Can you work these out from the model? Positions are in its coordinate system, mm. A direction names the side the tool comes from. Give positions to 0.01 mm unless a question says otherwise; leave off trailing zeros. Order: outer loops, then holes, each group sorted by start corner. A loop starts at its lowest first (then second) coordinate and runs counter-clockwise, first axis right, second up. Notation, with made-up numbers: M 34,42 L 84,42 A18 ccw 84,71 Z; hole C 72.25,-2.75 d9. An arc over 180 degrees is marked long. Write each question's results on one line, items separated by ' | '.
from build123d import *

# Parameters (mm, degrees)
CUT_EXTRUDE1_DEPTH = 1.41097
SKETCH5_R          = 1.833087105
CUT_EXTRUDE2_DEPTH = 1.41097
CUT_EXTRUDE2_DRAFT = -60
FILLET1_R          = 0.12827


with BuildPart() as part:
    # Sketch3 → Revolve1 (revolve)
    with BuildSketch(Plane(origin=(0, 0, 0), x_dir=(0, 0, -1), z_dir=(1, 0, 0))):
        with BuildLine():
            Line((-6.83895, 0), (-6.83895, 2.2225))
            ThreePointArc((-6.83895, 2.2225), (-5.93321038, 3.573966445), (-4.65836, 4.5847))
            Line((-4.65836, 4.5847), (-4.27355, 4.516847615))
            Line((-4.27355, 4.516847615), (-4.27355, 2.413))
            Line((-4.27355, 2.413), (6.2436375, 2.413))
            Line((6.2436375, 2.413), (6.83895, 1.8176875))
            Line((6.83895, 1.8176875), (6.83895, 0))
            Line((6.83895, 0), (-6.83895, 0))
        make_face()
    revolve(axis=Axis((0, 0, 6.83895), (0, 0, -1)))

    # Sketch4 → Cut-Extrude1 (cut)
    with BuildSketch(Plane.XY.offset(6.83895)):
        Polygon((-1.5875, -0.916543552), (0, -1.833087105), (1.5875, -0.916543552), (1.5875, 0.916543552), (0, 1.833087105), (-1.5875, 0.916543552), align=None)
    extrude(amount=-CUT_EXTRUDE1_DEPTH, mode=Mode.SUBTRACT)


with BuildPart() as cut_extrude2_tool:
    # Sketch5 → Cut-Extrude2 (with draft: the straight prism first)
    with BuildSketch(Plane.XY.offset(6.83895)):
        Circle(SKETCH5_R)
    extrude(amount=-CUT_EXTRUDE2_DEPTH)
    # Cut-Extrude2: the draft: its side faces are tilted about the plane it starts from
    cut_extrude2_sides = [cut_extrude2_tool.faces().sort_by_distance(p)[0] for p in [
        (-1.833087105, 0, 6.133465),
    ]]
    draft(cut_extrude2_sides, Plane.XY.offset(6.83895), CUT_EXTRUDE2_DRAFT)


with BuildPart() as part_1:
    add(part.part)

    # Cut-Extrude2: cut by cut_extrude2_tool
    add(cut_extrude2_tool.part, mode=Mode.SUBTRACT)

    # Fillet1
    fillet1_edges = [part_1.edges().sort_by_distance(p)[0] for p in [
        (0, -4.516847615, 4.27355),
        (0, -4.5847, 4.65836),
    ]]
    fillet(fillet1_edges, radius=FILLET1_R)


solid = part_1.part
(1) Imagine slicing it at B-B, the plane z = -1. Write out the boundary of the cut face in (x, y), plus the area to 3 significant figures.
Data:
outline: C 0,0 d4.83 | area: 18.3 mm2
(2) We'd pull the mould along Y, two halves only. Please class faces 1 (the face through (-1.588, 0, 6)), 2 (the face through (2, 0, 6.839)), 3 (the face through (-1.468, -1.915, -1.059)): +Y half, -Y half, draft (parallel to the pull), parting line (faces both ways), or undercut.
Data:
face 1: undercut | face 2: draft | face 3: parting line
(3) Imagine slicing it at A-A, the plane z = 5.75. Write out the boundary of the cut face in (x, y), plus the area to 3 significant figures.
Data:
outline: C 0,0 d7.53; hole M -1.59,-0.92 L 0,-1.83 L 1.59,-0.92 L 1.59,0.92 L 0,1.83 L -1.59,0.92 Z | area: 35.7 mm2
(4) For faces 4 (the face through (-2, 2, 4.274)), 5 (the face through (0, 0, -6.839)), 6 (the face through (0.8, 1.37, 6.14)), which set-ups out of +Z, -Z, +X, -X, +Y, -Y let a thin tool reach every point of the face, with its end or its side?
Data:
face 4: -Z | face 5: -Z, +X, -X, +Y, -Y | face 6: +Z
(5) I need wall thicknesses on L1, parallel to Z at x = 0, y = -1.75; L2, parallel to Z at x = 3.75, y = 0; L3, parallel to Y at x = 2.75, z = 5.75. Which ranges of each line are inside material? Lowest first, please. Write a range as from..to.
Data:
L1: z = -6.84..5.43 | L2: z = 4.27..5.76 | L3: y = -2.57..2.57
(6) Will these pins go through, and if not, where does the flat tip stop? P1, Ø4, axis at y = 1.5, z = 3, coming from the -X side; P2, Ø1.6, axis at x = 0.5, y = 0.5, coming from the +Z side; P3, Ø4, axis at x = -2, z = 0, coming from the -Y side.
Data:
P1: stops at x = -4.57 | P2: stops at z = 5.43 | P3: stops at y = -2.41
